Geometry check sheet. Reference: the model listing, model coordinates, mm. A direction names the side the tool comes from. Give positions to 0.01 mm unless a question says otherwise; leave off trailing zeros. Write each loop counter-clockwise with the first axis right and the second up, starting at its lowest first coordinate (ties: lowest second). Pieces come first, ordered by that corner, then holes. Notation, with made-up numbers: (48, 88) - (80, 88) arc R25 ccw to (80, 110) - close; hole circle Ø7 at (-28, 55). An arc over 180 degrees is marked (long way). One line per question, with ' | ' between items. Start each with the question number.
Q1. Thickness scan on L1, parallel to Y at x = 11.25, z = 22.2; L2, parallel to Y at x = 11, z = -13.5; L3, parallel to Y at x = 10.75, z = 15.7. Record the ranges inside material, lowest first. Write a range as [from, to].
Q2. Set-up check for faces 4 (the face through (9, -12, 27.325)), 5 (the face through (1.16, -2.955, -24.266)), 6 (the face through (11, -21.95, -15)), 7 (the face through (3.302, 18.757, -27.514)), 8 (the face through (1, -17, -18)): record each of +Z, -Z, +X, -X, +Y, -Y from which the full face is reachable in a straight line by a thin tool's end or side.
Q3. Section check D-D on x = 11.5. Count the separate pieces of the cut face and the enclosed holes in it, and give its area (3 significant figures).
Q4. Section check C-C on z = -5.5. Record the boundary of the cut face in (x, y), and give its area (3 significant figures).
Q5. Release check for a two-part mould opening along Y. For faces 1 (the face through (15, -19.85, 18)), 2 (the face through (1, -5, -25.85)), 3 (the face through (0, 5, 8)) record: +Y half, -Y half, draft (parallel to the pull), parting line (faces both ways), or undercut.
Q6. Gauge pin test, flat ends, axial feed: P1, Ø4, axis at x = 11.5, y = 11, coming from the -Z side (3 decimals); P2, Ø1.7, axis at x = 20.5, y = -20.5, coming from the +Z side (3 decimals); P3, Ø10, axis at y = -2.5, z = -11, coming from the +X side. Record the tip position at first contact, or that the pin passes through.
Q7. Section check A-A on z = -18.8. Record the boundary of the cut face in (x, y), and give its area (3 significant figures).
```python
from build123d import *

# Parameters (mm, degrees)
MAIN_EXTRUDE_DEPTH            = 2.2875
WALLS_START                   = 2.2875
WALLS_DEPTH                   = 13
CORNER_SUPPORT_DEPTH          = 2
SKETCH2_R                     = 0.95
SKETCH2_W                     = 2.4
SKETCH2_H                     = 4
SKETCH2_W_2                   = 1
SWITCH_SPACER_DEPTH           = 9.9
ARM_SUPPORT_EXTRUDE_DEPTH     = 3
ARM_SUPPORT_CURVE_DEPTH       = 40.380356778
FILLET4_R                     = 2
FILLET3_R                     = 2
SKETCH2_5_R                   = 0.95
SWITCH_MOUNT_HOLES_DEPTH      = 40.380356889
SWITCH_MOUNT_HOLES_DEPTH_BACK = 40.380356889
SKETCH35_R                    = 1.5
SWITCH_MOUNT_EXIT_HOLES_DEPTH = 3
SKETCH4_W                     = 8.5
SKETCH4_H                     = 5.5
WIRE_HOLE_DEPTH               = 40.380356889
SKETCH25_W                    = 6
SKETCH25_H                    = 1.35
FEMALE_SNAP_DEPTH             = 10.125
SKETCH5_W                     = 30
SKETCH5_H                     = 12.75
SERVO_HOLE_DEPTH              = 40.380356889
SKETCH30_W                    = 15.7875
SKETCH30_H                    = 0.9
SKETCH30_W_2                  = 17.7875
SKETCH30_H_2                  = 1.5
MAGNET_EXTRUDE_1_DEPTH        = 7.625
MAGNET_EXTRUDE_1_DEPTH_BACK   = 8.2
SKETCH30_5_W                  = 20.25
SKETCH30_5_H                  = 1.5
MAGNET_EXTRUDE_2_DEPTH        = 8.2
SKETCH29_R                    = 7.7
MAGNET_HOLE_DEPTH             = 2.1
SKETCH31_R                    = 5.5
MAGNET_THRU_HOLE_DEPTH        = 58.632218961


with BuildPart() as part:
    # Sketch1 → Main Extrude (new body)
    with BuildSketch(Plane(origin=(0, 0, 0), x_dir=(0, 0, -1), z_dir=(1, 0, 0))):
        Polygon((-30.5, -1.48), (-27.325, -1.48), (-27.325, -21.25), (28.5, -21.25), (28.5, 21.25), (-27.325, 21.25), (-27.325, 11.07), (-30.5, 11.07), align=None)
        with BuildLine():
            Line((20.7, 4.22), (-2.8, 4.22))
            ThreePointArc((-2.8, 4.22), (-4.6, 6.02), (-2.8, 7.82))
            Line((-2.8, 7.82), (20.7, 7.82))
            ThreePointArc((20.7, 7.82), (22.5, 6.02), (20.7, 4.22))
        make_face(mode=Mode.SUBTRACT)
    extrude(amount=MAIN_EXTRUDE_DEPTH)

    # Sketch1_3 → Walls (add)
    with BuildSketch(Plane(origin=(0, 0, 0), x_dir=(0, 0, -1), z_dir=(1, 0, 0)).offset(WALLS_START)):
        Polygon((-25.325, 19.25), (28.5, 19.25), (28.5, 21.25), (-27.325, 21.25), (-27.325, 11.07), (-30.5, 11.07), (-30.5, 9.17), (-25.325, 9.17), align=None)
        with BuildLine():
            Line((28.5, 2.445), (28, 2.445))
            ThreePointArc((28, 2.445), (26.939339828, 2.005660172), (26.5, 0.945))
            Line((26.5, 0.945), (26.5, -19.25))
            Line((26.5, -19.25), (-25.325, -19.25))
            Line((-25.325, -19.25), (-25.325, -0.23))
            Line((-25.325, -0.23), (-28.5, -0.23))
            Line((-28.5, -0.23), (-28.5, 3.42))
            Line((-28.5, 3.42), (-30.5, 3.42))
            Line((-30.5, 3.42), (-30.5, -1.48))
            Line((-30.5, -1.48), (-27.325, -1.48))
            Line((-27.325, -1.48), (-27.325, -21.25))
            Line((-27.325, -21.25), (28.5, -21.25))
            Line((28.5, -21.25), (28.5, 2.445))
        make_face()
    extrude(amount=WALLS_DEPTH)

    # Sketch22 → Corner Support (add)
    with BuildSketch(Plane(origin=(0, 0, -28.5), x_dir=(-1, 0, 0), z_dir=(0, 0, -1))):
        Polygon((-4.2875, 19.25), (-2.2875, 18.25), (-2.2875, 19.25), align=None)
    extrude(amount=-CORNER_SUPPORT_DEPTH)

    # Sketch2 → Switch Spacer (add)
    with BuildSketch(Plane(origin=(2.2875, 0, 0), x_dir=(0, 0, -1), z_dir=(1, 0, 0))):
        Polygon((-14.75, -2.88), (-17.75, -2.88), (-17.75, -6.88), (-14.75, -6.88), (-14.75, -4.88), align=None)
        with Locations((-15.7, -4.88)):
            Circle(SKETCH2_R, mode=Mode.SUBTRACT)
        with Locations((-15.7, -4.88)):
            Circle(SKETCH2_R)
        Polygon((-20.15, -2.88), (-23.15, -2.88), (-23.15, -4.88), (-23.15, -6.88), (-20.15, -6.88), align=None)
        with BuildLine():
            ThreePointArc((-21.25, -4.88), (-22.2, -5.83), (-23.15, -4.88))
            ThreePointArc((-23.15, -4.88), (-22.2, -3.93), (-21.25, -4.88))
        make_face(mode=Mode.SUBTRACT)
        with Locations((-22.2, -4.88)):
            Circle(SKETCH2_R)
        Polygon((-23.15, -4.88), (-23.15, -2.88), (-25.325, -2.88), (-25.325, -6.88), (-23.15, -6.88), align=None)
        with Locations((-18.95, -4.88)):
            Rectangle(SKETCH2_W, SKETCH2_H)
        with Locations((-14.25, -4.88)):
            Rectangle(SKETCH2_W_2, SKETCH2_H)
    extrude(amount=SWITCH_SPACER_DEPTH)

    # Sketch3 → Arm Support Extrude (add)
    with BuildSketch(Plane(origin=(2.2875, 0, 0), x_dir=(0, 0, -1), z_dir=(1, 0, 0))):
        with BuildLine():
            Line((-18.5, 5.62), (-10.5, 5.62))
            Line((-10.5, 5.62), (-10.5, 3.87))
            Line((-10.5, 3.87), (-28.5, 2.17))
            Line((-28.5, 2.17), (-30.5, 2.17))
            ThreePointArc((-30.5, 2.17), (-24.743046131, 4.740377849), (-18.5, 5.62))
        make_face()
    extrude(amount=ARM_SUPPORT_EXTRUDE_DEPTH)

    # Sketch7 → Arm Support Curve (cut, through all)
    with BuildSketch(Plane(origin=(2.2875, 0, 0), x_dir=(0, 0, -1), z_dir=(1, 0, 0))):
        with BuildLine():
            Line((-28.5, 3.286589176), (-28.5, 3.42))
            Line((-28.5, 3.42), (-30.5, 3.42))
            Line((-30.5, 3.42), (-30.5, 2.17))
            ThreePointArc((-30.5, 2.17), (-29.627655409, 2.689861102), (-28.73283292, 3.17))
            ThreePointArc((-28.73283292, 3.17), (-28.616584416, 3.228630003), (-28.5, 3.286589176))
        make_face()
    extrude(amount=ARM_SUPPORT_CURVE_DEPTH, mode=Mode.SUBTRACT)

    # Fillet4
    fillet4_edges = [part.edges().sort_by_distance(p)[0] for p in [
        (2.2875, 5.67, 30.5),
    ]]
    fillet(fillet4_edges, radius=FILLET4_R)

    # Fillet3
    fillet3_edges = [part.edges().sort_by_distance(p)[0] for p in [
        (2.2875, -6.88, 19.5375),
        (2.2875, -2.88, 19.5375),
    ]]
    fillet(fillet3_edges, radius=FILLET3_R)

    # Sketch2_5 → Switch Mount Holes (cut, two sides)
    with BuildSketch(Plane(origin=(2.2875, 0, 0), x_dir=(0, 0, -1), z_dir=(1, 0, 0))) as switch_mount_holes_sk:
        with Locations((-22.2, -4.88)):
            Circle(SKETCH2_5_R)
        with Locations((-15.7, -4.88)):
            Circle(SKETCH2_5_R)
    extrude(amount=SWITCH_MOUNT_HOLES_DEPTH, mode=Mode.SUBTRACT)
    extrude(switch_mount_holes_sk.sketch, amount=-SWITCH_MOUNT_HOLES_DEPTH_BACK, mode=Mode.SUBTRACT)

    # Sketch35 → Switch Mount Exit Holes (cut)
    with BuildSketch(Plane(origin=(12.1875, 0, 0), x_dir=(0, 0, -1), z_dir=(1, 0, 0))):
        with Locations((-22.2, -4.88)):
            Circle(SKETCH35_R)
        with Locations((-15.7, -4.88)):
            Circle(SKETCH35_R)
    extrude(amount=-SWITCH_MOUNT_EXIT_HOLES_DEPTH, mode=Mode.SUBTRACT)

    # Sketch4 → Wire Hole (cut, through all)
    with BuildSketch(Plane(origin=(2.2875, 0, 0), x_dir=(0, 0, -1), z_dir=(1, 0, 0))):
        with Locations((22.25, -16.5)):
            Rectangle(SKETCH4_W, SKETCH4_H)
    extrude(amount=-WIRE_HOLE_DEPTH, mode=Mode.SUBTRACT)

    # Sketch25 → Female Snap (cut, symmetric)
    with BuildSketch(Plane(origin=(0, 0, -0.5875), x_dir=(-1, 0, 0), z_dir=(0, 0, -1))):
        with Locations((-11.0375, -19.925)):
            Rectangle(SKETCH25_W, SKETCH25_H)
        Polygon((-15.2875, -19.25), (-15.2875, -19.91463679), (-14.0375, -19.25), align=None)
        with Locations((-11.0375, 19.925)):
            Rectangle(SKETCH25_W, SKETCH25_H)
        Polygon((-15.2875, 19.91463679), (-15.2875, 19.25), (-14.0375, 19.25), align=None)
    extrude(amount=FEMALE_SNAP_DEPTH, both=True, mode=Mode.SUBTRACT)

    # Sketch5 → Servo Hole (cut, through all)
    with BuildSketch(Plane(origin=(2.2875, 0, 0), x_dir=(0, 0, -1), z_dir=(1, 0, 0))):
        with Locations((6.65, -5.505)):
            Rectangle(SKETCH5_W, SKETCH5_H)
        with BuildLine():
            Line((-9.45, -4.505), (-9.45, -6.505))
            ThreePointArc((-9.45, -6.505), (-11, -8.055), (-12.55, -6.505))
            Line((-12.55, -6.505), (-12.55, -4.505))
            ThreePointArc((-12.55, -4.505), (-11, -2.955), (-9.45, -4.505))
        make_face()
        with BuildLine():
            Line((25.85, -4.505), (25.85, -6.505))
            ThreePointArc((25.85, -6.505), (24.3, -8.055), (22.75, -6.505))
            Line((22.75, -6.505), (22.75, -4.505))
            ThreePointArc((22.75, -4.505), (24.3, -2.955), (25.85, -4.505))
        make_face()
    extrude(amount=-SERVO_HOLE_DEPTH, mode=Mode.SUBTRACT)

    # Sketch30 → Magnet Extrude 1 (add, two sides)
    with BuildSketch(Plane(origin=(15.2875, 0, 0), x_dir=(0, 0, -1), z_dir=(1, 0, 0))) as magnet_extrude_1_sk:
        Polygon((-27.325, -18.35), (-27.325, -21.25), (-9.5375, -21.25), (-9.5375, -19.91463679), (-9.5375, -19.25), (-25.325, -19.25), (-25.325, -18.35), align=None)
        with Locations((-17.43125, -18.8)):
            Rectangle(SKETCH30_W, SKETCH30_H)
        with Locations((19.60625, -22)):
            Rectangle(SKETCH30_W_2, SKETCH30_H_2)
        Polygon((10.7125, -19.91463679), (10.7125, -21.25), (28.5, -21.25), (28.5, -18.35), (26.5, -18.35), (26.5, -19.25), (10.7125, -19.25), align=None)
        with Locations((-18.43125, -22)):
            Rectangle(SKETCH30_W_2, SKETCH30_H_2)
        with Locations((18.60625, -18.8)):
            Rectangle(SKETCH30_W, SKETCH30_H)
    extrude(amount=MAGNET_EXTRUDE_1_DEPTH)
    extrude(magnet_extrude_1_sk.sketch, amount=-MAGNET_EXTRUDE_1_DEPTH_BACK)

    # Sketch30_5 → Magnet Extrude 2 (add)
    with BuildSketch(Plane(origin=(15.2875, 0, 0), x_dir=(0, 0, -1), z_dir=(1, 0, 0))):
        with Locations((0.5875, -22)):
            Rectangle(SKETCH30_5_W, SKETCH30_5_H)
    extrude(amount=-MAGNET_EXTRUDE_2_DEPTH)

    # Sketch29 → Magnet Hole (cut)
    with BuildSketch(Plane(origin=(0, -21.95, 0), x_dir=(1, 0, 0), z_dir=(0, 1, 0))):
        with Locations((15.2875, -17.625)):
            Circle(SKETCH29_R)
        with BuildLine():
            ThreePointArc((22.9125, -18.697089082), (20.338980677, -23.436414885), (15.2875, -25.325))
            Line((15.2875, -25.325), (22.9125, -25.325))
            Line((22.9125, -25.325), (22.9125, -18.697089082))
        make_face()
        with BuildLine():
            Line((22.9125, -9.925), (15.2875, -9.925))
            ThreePointArc((15.2875, -9.925), (20.338980677, -11.813585115), (22.9125, -16.552910918))
            Line((22.9125, -16.552910918), (22.9125, -9.925))
        make_face()
        with Locations((15.2875, 18.8)):
            Circle(SKETCH29_R)
        with BuildLine():
            ThreePointArc((22.9125, 17.727910918), (20.338980677, 12.988585115), (15.2875, 11.1))
            Line((15.2875, 11.1), (22.9125, 11.1))
            Line((22.9125, 11.1), (22.9125, 17.727910918))
        make_face()
        with BuildLine():
            Line((22.9125, 26.5), (15.2875, 26.5))
            ThreePointArc((15.2875, 26.5), (20.338980677, 24.611414885), (22.9125, 19.872089082))
            Line((22.9125, 19.872089082), (22.9125, 26.5))
        make_face()
        with BuildLine():
            ThreePointArc((22.9875, -17.625), (22.968727116, -17.087645368), (22.9125, -16.552910918))
            Line((22.9125, -16.552910918), (22.9125, -18.697089082))
            ThreePointArc((22.9125, -18.697089082), (22.968727116, -18.162354632), (22.9875, -17.625))
        make_face()
        with BuildLine():
            Line((22.9125, 19.872089082), (22.9125, 17.727910918))
            ThreePointArc((22.9125, 17.727910918), (22.968727116, 18.262645368), (22.9875, 18.8))
            ThreePointArc((22.9875, 18.8), (22.968727116, 19.337354632), (22.9125, 19.872089082))
        make_face()
    extrude(amount=MAGNET_HOLE_DEPTH, mode=Mode.SUBTRACT)

    # Sketch31 → Magnet Thru Hole (cut, through all)
    with BuildSketch(Plane.XZ.offset(21.95)):
        with Locations((15.2875, 17.625)):
            Circle(SKETCH31_R)
        with BuildLine():
            Line((22.9125, 23.125), (15.2875, 23.125))
            ThreePointArc((15.2875, 23.125), (19.176587297, 21.514087297), (20.7875, 17.625))
            ThreePointArc((20.7875, 17.625), (19.176587297, 13.735912703), (15.2875, 12.125))
            Line((15.2875, 12.125), (22.9125, 12.125))
            Line((22.9125, 12.125), (22.9125, 23.125))
        make_face()
        with Locations((15.2875, -18.8)):
            Circle(SKETCH31_R)
        with BuildLine():
            Line((22.9125, -13.3), (15.2875, -13.3))
            ThreePointArc((15.2875, -13.3), (19.176587297, -14.910912703), (20.7875, -18.8))
            ThreePointArc((20.7875, -18.8), (19.176587297, -22.689087297), (15.2875, -24.3))
            Line((15.2875, -24.3), (22.9125, -24.3))
            Line((22.9125, -24.3), (22.9125, -13.3))
        make_face()
    extrude(amount=MAGNET_THRU_HOLE_DEPTH, mode=Mode.SUBTRACT)


solid = part.part
```
Working result:
1) L1: y = [-22.75, -21.95], [-19.85, -18.35], [-6.88, -6.38], [-3.38, -2.88], [19.25, 21.25] | L2: y = [-22.75, -21.95], [-19.85, -18.35], [19.25, 21.25] | L3: y = [-19.85, -18.35], [-6.88, -6.38], [-3.38, -2.88], [19.25, 21.25]
2) face 4: +Z, +X, -X, -Y | face 5: +X, -X | face 6: +X | face 7: -Z, +X | face 8: -X
3) separate pieces: 2 | enclosed holes: 2 | area: 361 mm2
4) outline: (0, -21.25) - (7.09, -21.25) - (7.09, -22.75) - (15.29, -22.75) - (15.29, -19.91) - (14.04, -19.25) - (14.04, -20.6) - (8.04, -20.6) - (8.04, -19.25) - (2.29, -19.25) - (2.29, -11.88) - (0, -11.88) - close; (0, 0.87) - (2.29, 0.87) - (2.29, 4.22) - (0, 4.22) - close; (0, 7.82) - (2.29, 7.82) - (2.29, 19.25) - (8.04, 19.25) - (8.04, 20.6) - (14.04, 20.6) - (14.04, 19.25) - (15.29, 19.91) - (15.29, 21.25) - (0, 21.25) - close | area: 107 mm2
5) face 1: undercut | face 2: undercut | face 3: draft
6) P1: stops at z = 25.325 | P2: stops at z = 27.325 | P3: stops at x = 2.29
7) outline: (0, -21.25) - (7.09, -21.25) - (7.09, -22.75) - (9.79, -22.75) - (9.79, -21.95) - (7.59, -21.95) - (7.59, -19.85) - (22.91, -19.85) - (22.91, -18.35) - (7.09, -18.35) - (7.09, -19.25) - (0, -19.25) - close; (0, -13.75) - (2.29, -13.75) - (2.29, -11.88) - (0, -11.88) - close; (0, 0.87) - (2.29, 0.87) - (2.29, 4.22) - (0, 4.22) - close; (0, 7.82) - (2.29, 7.82) - (2.29, 19.25) - (15.29, 19.25) - (15.29, 21.25) - (0, 21.25) - close | area: 110 mm2
